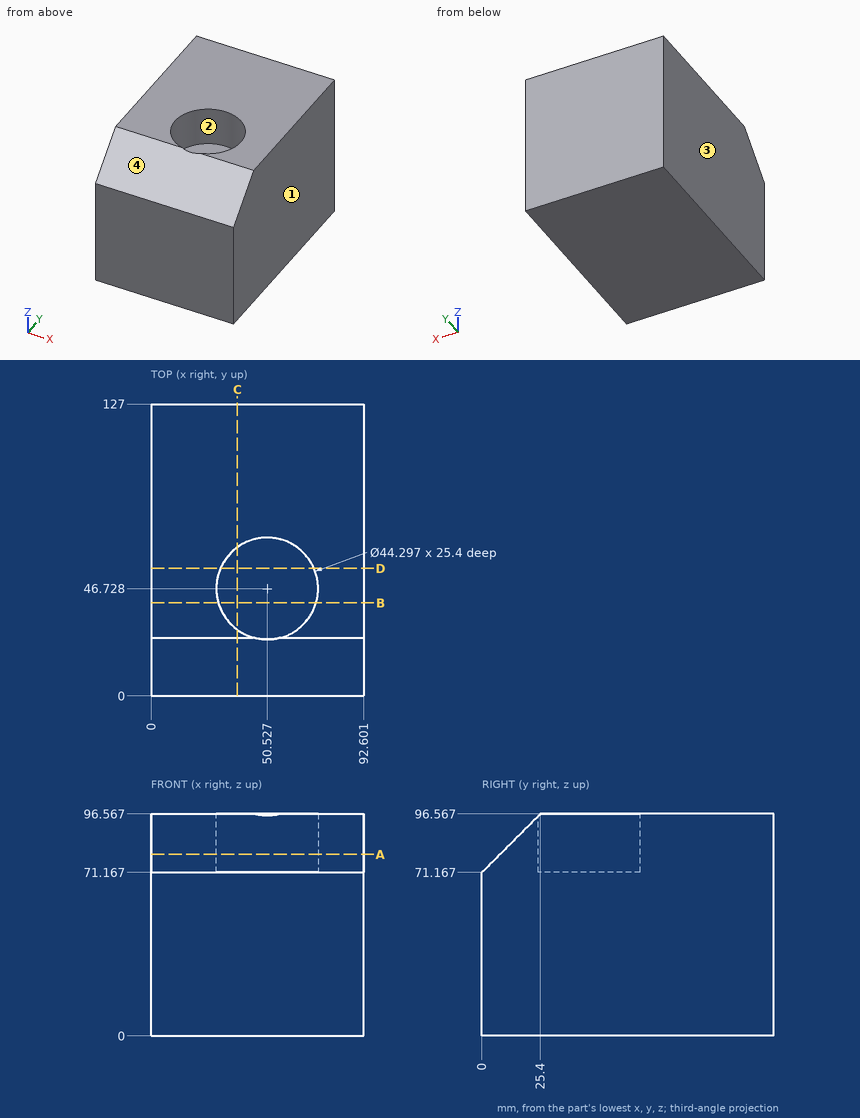
Design review of the part shown in the three views and the two pictorial views. Dimensions are in mm from the part's minimum x, y and z. Coordinates: 2 decimals unless noted, no trailing zeros. Write each loop counter-clockwise with the first axis right and the second up, starting at its lowest first coordinate (ties: lowest second). Pieces come first, ordered by that corner, then holes.
1) We need section C-C on x = 37.5. State the section outline as (y, z) points, then the cut area to 3 significant figures.
2) The part is to be moulded in two halves that separate along X. For the marked faces 1, 2, 3 and 4, say which applies: pulls with the +X half, pulls with the -X half, needs draft (parallel to the pull), parting line crosses it, or undercut.
3) We need section B-B on y = 40.5. State the section outline as (x, z) points, then the cut area to 3 significant figures.
4) We need section A-A on z = 79. State the section outline as (x, y) points (1 decimal).
5) We need section D-D on y = 55.5. State the section outline as (x, z) points (1 decimal), then the cut area to 3 significant figures.
6) To check wall thickness, follow probe 1 along Z at (x, y) = (47.5, 30.5); probe 2 along X at (y, z) = (45, 81.5); probe 3 along Z at (x, y) = (33, 9) (1 decimal). State the ranges of each line that lie inside material, in increasing order.
Answer list:
1. outline: (0, 0) - (127, 0) - (127, 96.57) - (64.64, 96.57) - (64.64, 71.17) - (28.82, 71.17) - (28.82, 96.57) - (25.4, 96.57) - (0, 71.17) - close
1. area: 11,000 mm2
2. face 1: pulls with the +X half
2. face 2: undercut
2. face 3: pulls with the -X half
2. face 4: needs draft
3. outline: (0, 0) - (92.6, 0) - (92.6, 96.57) - (71.78, 96.57) - (71.78, 71.17) - (29.27, 71.17) - (29.27, 96.57) - (0, 96.57) - close
3. area: 7,860 mm2
4. outline: (0, 7.8) - (92.6, 7.8) - (92.6, 127) - (0, 127) - close; hole circle Ø44.3 at (50.5, 46.7)
5. outline: (0, 0) - (92.6, 0) - (92.6, 96.6) - (70.9, 96.6) - (70.9, 71.2) - (30.2, 71.2) - (30.2, 96.6) - (0, 96.6) - close
5. area: 7,910 mm2
6. probe 1: z = 0 to 71.17
6. probe 2: x = 0 to 28.45, 72.61 to 92.6
6. probe 3: z = 0 to 80.2
